```python
from build123d import *

# Parameters (mm, degrees)
BOSS_EXTRUDE1_DEPTH              = 3.175
FILLET1_R                        = 3.175
F_1_4_0_25_DIAMETER_HOLE1_D      = 6.35
F_17_64_0_26563_DIAMETER_HOLE1_D = 6.747002
SKETCH9_R                        = 3.175
CUT_EXTRUDE1_DEPTH               = 425.763278612


with BuildPart() as part:
    # Sketch1 → Boss-Extrude1 (new body)
    with BuildSketch(Plane(origin=(0, 0, 0), x_dir=(1, 0, 0), z_dir=(0, 1, 0))):
        Polygon((0, 0), (273.05, 0), (273.05, 19.05), (336.55, 260.35), (0, 260.35), align=None)
    extrude(amount=BOSS_EXTRUDE1_DEPTH)

    # Fillet1
    fillet1_edges = [part.edges().sort_by_distance(p)[0] for p in [
        (0, 1.5875, -260.35),
        (336.55, 1.5875, -260.35),
        (273.05, 1.5875, -19.05),
        (273.05, 1.5875, 0),
        (0, 1.5875, 0),
    ]]
    fillet(fillet1_edges, radius=FILLET1_R)

    # 1/4 (0.25) Diameter Hole1 (through all)
    with Locations(Plane(origin=(0, 3.175, 0), x_dir=(1, 0, 0), z_dir=(0, 1, 0))):
        with Locations((43.97818809, 254), (170.97818809, 254), (297.97818809, 254), (311.721536551, 190.953379927), (279.400887542, 68.134913694)):
            Hole(F_1_4_0_25_DIAMETER_HOLE1_D / 2)

    # 17/64 (0.26563) Diameter Hole1 (through all)
    with Locations(Plane(origin=(0, 3.175, 0), x_dir=(1, 0, 0), z_dir=(0, 1, 0))):
        with Locations((12.7, 9.525), (139.7, 9.525)):
            Hole(F_17_64_0_26563_DIAMETER_HOLE1_D / 2)

    # Sketch9 → Cut-Extrude1 (cut, through all)
    with BuildSketch(Plane(origin=(0, 3.175, 0), x_dir=(1, 0, 0), z_dir=(0, 1, 0))):
        with Locations(Location((297.97818809, 254, 0), (0, 0, 270))):
            Circle(SKETCH9_R)
        with Locations(Location((170.97818809, 254, 0), (0, 0, 270))):
            Circle(SKETCH9_R)
        with Locations(Location((43.97818809, 254, 0), (0, 0, 270))):
            Circle(SKETCH9_R)
        with BuildLine():
            Line((31.27818809, 244.475), (56.67818809, 244.475))
            ThreePointArc((56.67818809, 244.475), (66.20318809, 234.95), (56.67818809, 225.425))
            Line((56.67818809, 225.425), (31.27818809, 225.425))
            ThreePointArc((31.27818809, 225.425), (21.75318809, 234.95), (31.27818809, 244.475))
        make_face()
        with BuildLine():
            Line((158.27818809, 244.475), (183.67818809, 244.475))
            ThreePointArc((183.67818809, 244.475), (193.20318809, 234.95), (183.67818809, 225.425))
            Line((183.67818809, 225.425), (158.27818809, 225.425))
            ThreePointArc((158.27818809, 225.425), (148.75318809, 234.95), (158.27818809, 244.475))
        make_face()
        with BuildLine():
            Line((285.27818809, 244.475), (310.67818809, 244.475))
            ThreePointArc((310.67818809, 244.475), (320.20318809, 234.95), (310.67818809, 225.425))
            Line((310.67818809, 225.425), (285.27818809, 225.425))
            ThreePointArc((285.27818809, 225.425), (275.75318809, 234.95), (285.27818809, 244.475))
        make_face()
    extrude(amount=-CUT_EXTRUDE1_DEPTH, mode=Mode.SUBTRACT)


solid = part.part
```
Work out the finished part from the listing and answer in its coordinate system (mm). A direction names the side the tool comes from. Give positions to 0.01 mm unless a question says otherwise; leave off trailing zeros. Loops run counter-clockwise (first coordinate to the right, second up) from the corner with the lowest first, then second, coordinate; pieces in that order, holes last. Notation, with made-up numbers: (55.25, -10.5) -> (87.25, -10.5) arc R25 cw to (87.25, 27.5) -> close; hole circle Ø3 at (26, 55). An arc over 180 degrees is marked (long way). Use CSV: the item, a comma, the result in double quotes.
1. The part is cut by section C-C (y = 1.65). State how many separate pieces and enclosed holes the cut face has, then the cut area to 3 significant figures.
Found:
separate pieces,"1"
enclosed holes,"10"
area,"76,200 mm^2"
2. The part is cut by section A-A (x = 178.5). Write down the section's boundary in (y, z) (3 decimals), then the cut area to 3 significant figures.
Found:
outline,"(0, -260.35) -> (3.175, -260.35) -> (3.175, -244.475) -> (0, -244.475) -> close; (0, -225.425) -> (3.175, -225.425) -> (3.175, 0) -> (0, 0) -> close"
area,"766 mm^2"
3. The part is cut by section B-B (z = -229.5). Write down the section's boundary in (x, y) (3 decimals), then the cut area to 3 significant figures.
Found:
outline,"(0, 0) -> (23.466, 0) -> (23.466, 3.175) -> (0, 3.175) -> close; (64.49, 0) -> (150.466, 0) -> (150.466, 3.175) -> (64.49, 3.175) -> close; (191.49, 0) -> (277.466, 0) -> (277.466, 3.175) -> (191.49, 3.175) -> close; (318.49, 0) -> (328.432, 0) -> (328.432, 3.175) -> (318.49, 3.175) -> close"
area,"652 mm^2"
4. The mould has two halves that part along X. Classify faces 3 (the flat face through (303.892, 1.565, -136.249)), 4 (the flat face through (165, 0, -132)), 5 (the cylindrical face through (66.2, 1.6, -235.2)): +X half, -X half, draft (parallel to the pull), parting line (faces both ways), or undercut.
Found:
face 3,"+X half"
face 4,"draft"
face 5,"undercut"
5. The part is cut by section D-D (z = -87). Write down the section's boundary in (x, y) (3 decimals), then the cut area to 3 significant figures.
Found:
outline,"(0, 0) -> (290.932, 0) -> (290.932, 3.175) -> (0, 3.175) -> close"
area,"924 mm^2"
6. A tool of negligible diameter and unlimited length cuts with its end or side. For faces 1 (the flat face through (165, 3.175, -132)), 2 (the cylindrical face through (193.2, 1.6, -235.2)), from which of +Z, -Z, +X, -X, +Y, -Y can it reach the whole face along a straight path? Write none if from no direction.
Found:
face 1,"+Z, -Z, +X, -X, +Y"
face 2,"+Y, -Y"
7. A flat-ended cylindrical pin translates along its axis: pin 1 Ø4 at (x, z) = (170.98, -254) entering from +Y. Find the tip coordinate at first contact, or state that the pin passes through.
Found:
pin 1,"through"
8. Straight lines are drawn through the part: line 1 (Z direction, x = 12.7, y = 2.35); line 2 (Z direction, x = 139, y = 0.5); line 3 (X direction, y = 1.95, z = -233). For each, find the intervals that lie inside material, in ascending order.
Found:
line 1,"-260.35 to -12.9, -6.15 to 0"
line 2,"-260.35 to -12.83, -6.22 to 0"
line 3,"0 to 21.95, 66 to 148.95, 193 to 275.95, 320 to 329.35"
